For this review, take the finished solid that the model builds, in its own axes (mm). A direction names the side the tool comes from. Give positions to 0.01 mm unless a question says otherwise; leave off trailing zeros. Write each loop counter-clockwise with the first axis right and the second up, starting at its lowest first coordinate (ties: lowest second). Pieces come first, ordered by that corner, then holes.
1) Draft analysis for pull direction Z (two halves, no side actions). For faces 1 (the face through (-0.9, 0.054, -7.794)), 2 (the face through (3, -3, 30)), 3 (the face through (0, 0, -10)), state which applies: pulls with the +Z half, pulls with the -Z half, needs draft (parallel to the pull), parting line crosses it, or undercut.
2) We need section A-A on y = -2.5. Give the boundary of the cut face in (x, z), and give its area (3 significant figures).
3) We need section B-B on z = 10. Give the boundary of the cut face in (x, y), and give its area (3 significant figures).
4) We need section D-D on z = 0.5. Give the boundary of the cut face in (x, y).
5) Wall thickness on line 1 along X through (y, z) = (0.25, 3.5); line 2 along Z through (x, y) = (0, 4.75); line 3 along Y through (x, z) = (0, 14.25): over which ranges is each line inside the solid? List them lowest first.
6) We need section C-C on x = -2.25. Give the boundary of the cut face in (y, z), and give its area (3 significant figures).
7) For P1, Ø2.5, axis at x = 0, y = -1, coming from the +Z side; P2, Ø2, axis at x = 1, z = -4, coming from the +Y side; P3, Ø2, axis at y = -2, z = 15.5, coming from the +X side; P4, Ø1.8, axis at x = -0.29, z = -7, coming from the +Y side, all flat-tipped, find the tip position at first contact; note any pin that passes through.
8) Machinability: for faces 4 (the face through (3, -3, 0)), 5 (the face through (-0.867, -3.905, 17.675)), 6 (the face through (-1.46, -6.59, 14.79)), which of the approach directions +Z, -Z, +X, -X, +Y, -Y give a long, thin tool a straight path to every point of the face, cutting with its end or side? Answer none if there is none.
from build123d import *

# Parameters (mm, degrees)
SKETCH1_R           = 6.75
BOSS_EXTRUDE1_DEPTH = 30
SKETCH3_R           = 4
BOSS_EXTRUDE4_DEPTH = 10
SKETCH4_R           = 1
CUT_EXTRUDE2_DEPTH  = 15
SKETCH2_R           = 4
CUT_EXTRUDE3_DEPTH  = 25


with BuildPart() as part:
    # Sketch1 → Boss-Extrude1 (new body)
    with BuildSketch(Plane.XY):
        Circle(SKETCH1_R)
    extrude(amount=BOSS_EXTRUDE1_DEPTH)

    # Sketch3 → Boss-Extrude4 (add)
    with BuildSketch(Plane(origin=(0, 0, 0), x_dir=(-1, 0, 0), z_dir=(0, 0, -1))):
        with Locations(Location((0, 0, 0), (0, 0, 180))):
            Circle(SKETCH3_R)
    extrude(amount=BOSS_EXTRUDE4_DEPTH)

    # Sketch4 → Cut-Extrude2 (cut)
    with BuildSketch(Plane(origin=(0, 4, 0), x_dir=(1, 0, 0), z_dir=(0, 1, 0))):
        with Locations(Location((-0.291407977, 7, 0), (0, 0, 270))):
            Circle(SKETCH4_R)
    extrude(amount=-CUT_EXTRUDE2_DEPTH, mode=Mode.SUBTRACT)

    # Sketch2 → Cut-Extrude3 (cut)
    with BuildSketch(Plane.XY.offset(30)):
        Circle(SKETCH2_R)
    extrude(amount=-CUT_EXTRUDE3_DEPTH, mode=Mode.SUBTRACT)


solid = part.part
Results list:
1. face 1: undercut
1. face 2: pulls with the +Z half
1. face 3: pulls with the -Z half
2. outline: (-6.27, 0) - (-3.12, 0) - (-3.12, -10) - (3.12, -10) - (3.12, 0) - (6.27, 0) - (6.27, 30) - (3.12, 30) - (3.12, 5) - (-3.12, 5) - (-3.12, 30) - (-6.27, 30) - close; hole circle Ø2 at (-0.29, -7)
2. area: 279 mm2
3. outline: circle Ø13.5 at (0, 0); hole circle Ø8 at (0, 0)
3. area: 92.9 mm2
4. outline: circle Ø13.5 at (0, 0)
5. line 1: x = -6.75 to 6.75
5. line 2: z = 0 to 30
5. line 3: y = -6.75 to -4, 4 to 6.75
6. outline: (-6.36, 0) - (-3.31, 0) - (-3.31, -10) - (3.31, -10) - (3.31, 0) - (6.36, 0) - (6.36, 30) - (3.31, 30) - (3.31, 5) - (-3.31, 5) - (-3.31, 30) - (-6.36, 30) - close
6. area: 283 mm2
7. P1: stops at z = 5
7. P2: stops at y = 4
7. P3: stops at x = 6.68
7. P4: passes through
8. face 4: -Z
8. face 5: +Z
8. face 6: +Z, -Z
